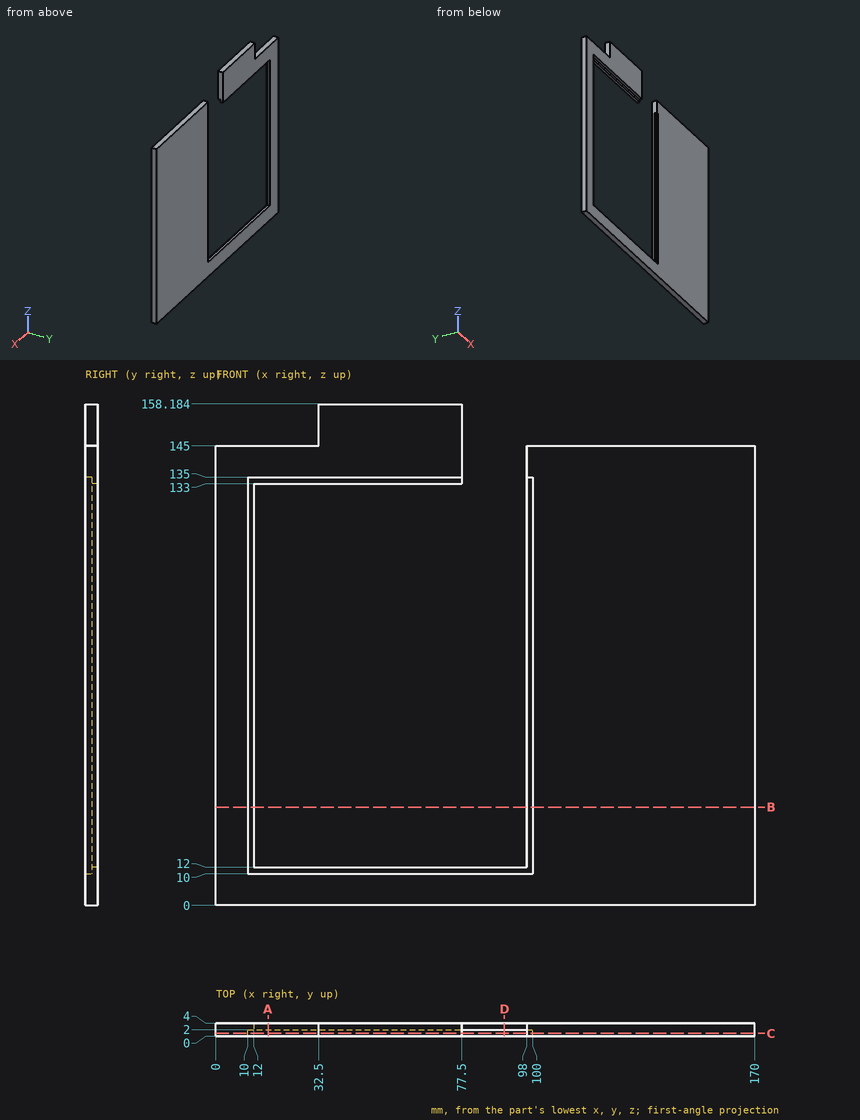
Part print with two shaded views. Sizes in mm from the minimum x, y, z corner. Round coordinates to 2 decimals unless told otherwise and drop trailing zeros. Order: outer loops, then holes, each group sorted by start corner. A loop starts at its lowest first (then second) coordinate and runs counter-clockwise, first axis right, second up. Notation, with made-up numbers: M 51.5,-30 L 79.5,-30 A33 ccw 79.5,9 Z; hole C 67.5,5 d5. An arc over 180 degrees is marked long. Answer in a Markdown table with one row per item. Add a question column.
Q1. Pin check, flat tips, straight feed: pin 1 (2 mm diameter, centred on x = 16, y = 1, fed in from +Z); pin 2 (2 mm diameter, centred on y = 1.5, z = 148.5, fed in from -X). Stop position of each tip, or through.
Q2. Cut at D-D on x = 91. Give the cut face in (y, z).
Q3. Wall check: L1, parallel to Z at x = 27.5, y = 1.15; L2, parallel to X at y = 3.55, z = 82; L3, parallel to X at y = 1.9, z = 33.5. Give the ranges that are in metal, low to high. Write a range as from..to.
Q4. Cut at C-C on y = 0.8. Give the cut face in (x, z), and give its area (3 significant figures).
Q5. Cut at B-B on z = 31. Give the cut face in (x, y).
Q6. Cut at A-A on x = 16.5. Give the cut face in (y, z), and give its area (3 significant figures).
Established:
| question | item | result |
|---|---|---|
| 1 | pin 1 | stops at z = 145 |
| 1 | pin 2 | stops at x = 32.5 |
| 2 | outline | M 0,0 L 4,0 L 4,12 L 2,12 L 2,10 L 0,10 Z |
| 3 | L1 | z = 0..10, 135..145 |
| 3 | L2 | x = 0..12, 98..170 |
| 3 | L3 | x = 0..10, 100..170 |
| 4 | outline | M 0,0 L 170,0 L 170,145 L 98,145 L 98,135 L 100,135 L 100,10 L 10,10 L 10,135 L 77.5,135 L 77.5,158.18 L 32.5,158.18 L 32.5,145 L 0,145 Z |
| 4 | area | 13,800 mm2 |
| 5 | outline | M 0,0 L 10,0 L 10,2 L 12,2 L 12,4 L 0,4 Z; M 98,2 L 100,2 L 100,0 L 170,0 L 170,4 L 98,4 Z |
| 6 | outline | M 0,0 L 4,0 L 4,12 L 2,12 L 2,10 L 0,10 Z; M 0,135 L 2,135 L 2,133 L 4,133 L 4,145 L 0,145 Z |
| 6 | area | 88.0 mm2 |
